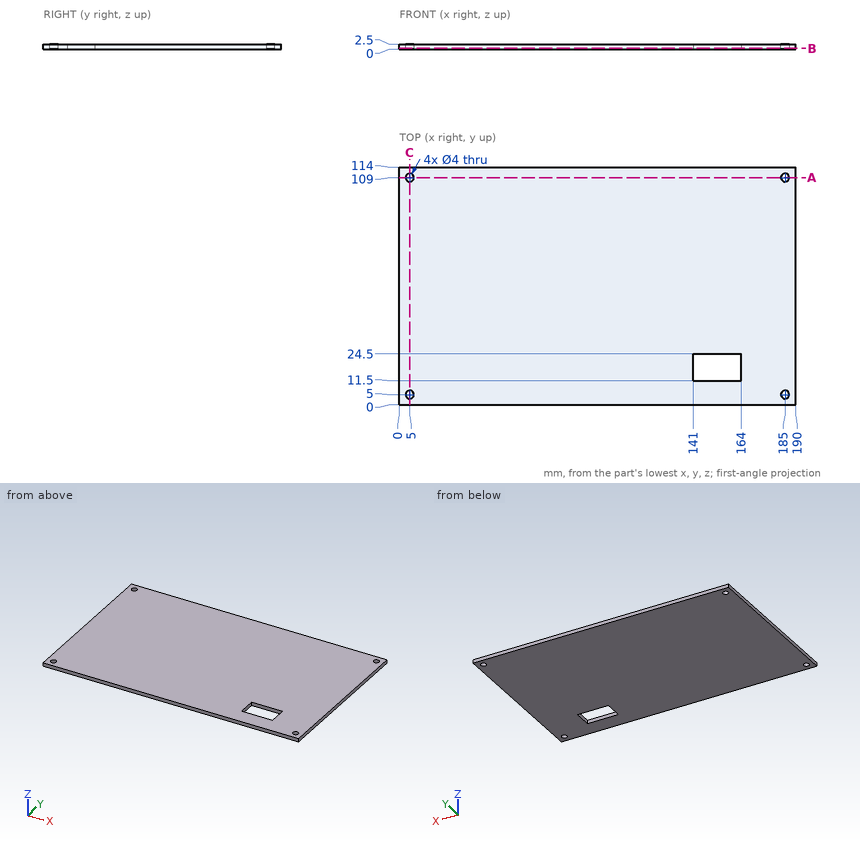
Geometry check sheet. Reference: drawing and pictorial views, mm from the part's lowest x, y, z. Round coordinates to 2 decimals unless told otherwise and drop trailing zeros. Order: outer loops, then holes, each group sorted by start corner. A loop starts at its lowest first (then second) coordinate and runs counter-clockwise, first axis right, second up. Notation, with made-up numbers: M 42.25,-34.75 L 63.25,-34.75 A29 ccw 63.25,-11.75 Z; hole C 82.25,18.25 d7. An arc over 180 degrees is marked long. One line per item, written item: value. Start each with the question number.
1. Section check A-A on y = 109. Enter the section's corners in (x, z), and give its area (3 significant figures).
2. Section check B-B on z = 0.4. Enter the section's corners in (x, y).
3. Scan lines: line 1 along Y through (x, z) = (5, 1.8); line 2 along X through (y, z) = (109, 1.25); line 3 along X through (y, z) = (21, 1.1). Record each from-to range of solid material in increasing order.
4. Section check C-C on x = 5. Enter the section's corners in (y, z).
Results found:
1. outline: M 0,0 L 3,0 L 3,2.5 L 0,2.5 Z; M 7,0 L 183,0 L 183,2.5 L 7,2.5 Z; M 187,0 L 190,0 L 190,2.5 L 187,2.5 Z
1. area: 455 mm^2
2. outline: M 0,0 L 190,0 L 190,114 L 0,114 Z; hole C 5,5 d4; hole C 5,109 d4; hole M 141,11.5 L 164,11.5 L 164,24.5 L 141,24.5 Z; hole C 185,5 d4; hole C 185,109 d4
3. line 1: 0 to 3, 7 to 107, 111 to 114
3. line 2: 0 to 3, 7 to 183, 187 to 190
3. line 3: 0 to 141, 164 to 190
4. outline: M 0,0 L 3,0 L 3,2.5 L 0,2.5 Z; M 7,0 L 107,0 L 107,2.5 L 7,2.5 Z; M 111,0 L 114,0 L 114,2.5 L 111,2.5 Z
